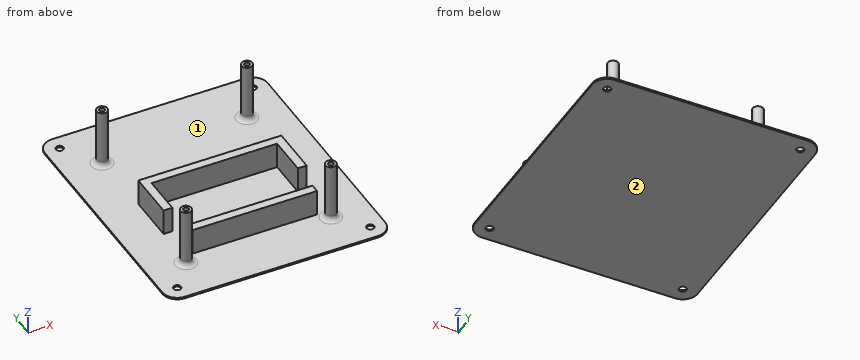
```python
from build123d import *

# Parameters (mm, degrees)
BASE_FLANGE1_DEPTH      = 1
SKETCH7_R               = 2.125
CUT_EXTRUDE1_DEPTH      = 10
SKETCH8_R               = 3
BOSS_EXTRUDE3_DEPTH     = 34
EXTRUDE_THIN1_OUTLINE_W = 71
EXTRUDE_THIN1_OUTLINE_H = 5
EXTRUDE_THIN1_DEPTH     = 15
SKETCH17_R              = 1.5
CUT_EXTRUDE3_DEPTH      = 13
SKETCH15_R              = 1.5
CUT_EXTRUDE4_DEPTH      = 13
SKETCH13_R              = 1.5
CUT_EXTRUDE5_DEPTH      = 13
SKETCH14_R              = 1.5
CUT_EXTRUDE6_DEPTH      = 13
FILLET1_R               = 3
FILLET2_R               = 3
FILLET3_R               = 3
FILLET4_R               = 3


# Read off the part's stored shape, not the designer's step: Extrude-Thin1
# Sheet-metal steps are written as plain solids
with BuildPart() as part:
    # Sketch1 → Base-Flange1 (new body)
    with BuildSketch(Plane.XY):
        with BuildLine():
            Line((-55.005, -73.465), (55.005, -73.465))
            ThreePointArc((55.005, -73.465), (60.987123369, -70.987123369), (63.465, -65.005))
            Line((63.465, -65.005), (63.465, 65.005))
            ThreePointArc((63.465, 65.005), (60.987123369, 70.987123369), (55.005, 73.465))
            Line((55.005, 73.465), (-55.005, 73.465))
            ThreePointArc((-55.005, 73.465), (-60.987123369, 70.987123369), (-63.465, 65.005))
            Line((-63.465, 65.005), (-63.465, -65.005))
            ThreePointArc((-63.465, -65.005), (-60.987123369, -70.987123369), (-55.005, -73.465))
        make_face()
    extrude(amount=-BASE_FLANGE1_DEPTH)

    # Sketch7 → Cut-Extrude1 (cut)
    with BuildSketch(Plane(origin=(0, 0, -1), x_dir=(-1, 0, 0), z_dir=(0, 0, -1))):
        with Locations((55.005, 65.005)):
            Circle(SKETCH7_R)
        with Locations((-55.005, 65.005)):
            Circle(SKETCH7_R)
        with Locations((55.005, -65.005)):
            Circle(SKETCH7_R)
        with Locations((-55.005, -65.005)):
            Circle(SKETCH7_R)
    extrude(amount=-CUT_EXTRUDE1_DEPTH, mode=Mode.SUBTRACT)

    # Sketch8 → Boss-Extrude3 (add)
    with BuildSketch(Plane.XY):
        with Locations((-41.5, -48.465)):
            Circle(SKETCH8_R)
        with Locations((-41.5, 44.372)):
            Circle(SKETCH8_R)
        with Locations((41.05, -48.465)):
            Circle(SKETCH8_R)
        with Locations((41.05, 44.372)):
            Circle(SKETCH8_R)
    extrude(amount=BOSS_EXTRUDE3_DEPTH)

    # Extrude-Thin1 outline → Extrude-Thin1 (add)
    with BuildSketch(Plane.XY):
        with Locations((0.25, -40.965)):
            Rectangle(EXTRUDE_THIN1_OUTLINE_W, EXTRUDE_THIN1_OUTLINE_H)
        Polygon((-40.75, 5.735), (-40.75, -22.265), (-35.75, -22.265), (-35.75, 0.735), (35.75, 0.735), (35.75, -22.265), (40.75, -22.265), (40.75, 5.735), align=None)
    extrude(amount=EXTRUDE_THIN1_DEPTH)

    # Sketch17 → Cut-Extrude3 (cut)
    with BuildSketch(Plane.XY.offset(34)):
        with Locations((41.05, -48.465)):
            Circle(SKETCH17_R)
    extrude(amount=-CUT_EXTRUDE3_DEPTH, mode=Mode.SUBTRACT)

    # Sketch15 → Cut-Extrude4 (cut)
    with BuildSketch(Plane.XY.offset(34)):
        with Locations((-41.5, -48.465)):
            Circle(SKETCH15_R)
    extrude(amount=-CUT_EXTRUDE4_DEPTH, mode=Mode.SUBTRACT)

    # Sketch13 → Cut-Extrude5 (cut)
    with BuildSketch(Plane.XY.offset(34)):
        with Locations((-41.5, 44.372)):
            Circle(SKETCH13_R)
    extrude(amount=-CUT_EXTRUDE5_DEPTH, mode=Mode.SUBTRACT)

    # Sketch14 → Cut-Extrude6 (cut)
    with BuildSketch(Plane.XY.offset(34)):
        with Locations((41.05, 44.372)):
            Circle(SKETCH14_R)
    extrude(amount=-CUT_EXTRUDE6_DEPTH, mode=Mode.SUBTRACT)

    # Fillet1
    fillet1_edges = [part.edges().sort_by_distance(p)[0] for p in [
        (-44.5, -48.465, 0),
    ]]
    fillet(fillet1_edges, radius=FILLET1_R)

    # Fillet2
    fillet2_edges = [part.edges().sort_by_distance(p)[0] for p in [
        (38.05, -48.465, 0),
    ]]
    fillet(fillet2_edges, radius=FILLET2_R)

    # Fillet3
    fillet3_edges = [part.edges().sort_by_distance(p)[0] for p in [
        (-44.5, 44.372, 0),
    ]]
    fillet(fillet3_edges, radius=FILLET3_R)

    # Fillet4
    fillet4_edges = [part.edges().sort_by_distance(p)[0] for p in [
        (38.05, 44.372, 0),
    ]]
    fillet(fillet4_edges, radius=FILLET4_R)


solid = part.part
```
Here's how the part is built. I have some questions about the finished solid (model axes, mm). Face numbers are marked on the shaded views. Give positions to 0.01 mm unless a question says otherwise; leave off trailing zeros. Order: outer loops, then holes, each group sorted by start corner. A loop starts at its lowest first (then second) coordinate and runs counter-clockwise, first axis right, second up. Notation, with made-up numbers: (12.5, 23.5) - (36.5, 23.5) arc R8 ccw to (36.5, 37.5) - close; hole circle Ø8 at (66.5, 7.25). An arc over 180 degrees is marked (long way). Answer as a JSON object with one key per item and string values. Group by question number.
Item 1: If we section it at B-B on y = -9: Please give me the cut outline in (x, z) (3 decimals).
Item 2: If we section it at A-A on z = 24.5: Please give me the cut outline in (x, y) (3 decimals).
Item 3: For P1, Ø0.9, axis at x = 41.5, y = 44, coming from the +Z side; P2, Ø7.5, axis at x = -14.5, z = 5, coming from the +Y side (3 decimals); P3, Ø12, axis at x = 19.5, y = 29.5, coming from the +Z side, each with a flat end and sliding along its axis, tell me the tip position at first contact or that it passes through.
Item 4: If we section it at D-D on y = -28.5: Please give me the cut outline in (x, z) (3 decimals).
Item 5: If we section it at C-C on z = 12.5: Please give me the cut outline in (x, y) (3 decimals).
Item 6: Please list where these lines run through material, in increasing order: probe 1 along Y at (x, z) = (41.05, 30) (3 decimals); probe 2 along Y at (x, z) = (-19.5, 14) (3 decimals); probe 3 along Z at (x, y) = (-14.5, 52.5).
Item 7: If we mould it in two halves opening along X, with no side actions, what happens to the marked faces 1 and 2? For each: pulls with the +X half, pulls with the -X half, needs draft (parallel to the pull), parting line crosses it, or undercut.
Result set:
{
 "1": {"outline": "(-63.465, -1) - (63.465, -1) - (63.465, 0) - (40.75, 0) - (40.75, 15) - (35.75, 15) - (35.75, 0) - (-35.75, 0) - (-35.75, 15) - (-40.75, 15) - (-40.75, 0) - (-63.465, 0) - close"},
 "2": {"outline": "circle Ø6 at (-41.5, -48.465); circle Ø6 at (-41.5, 44.372); circle Ø6 at (41.05, -48.465); circle Ø6 at (41.05, 44.372); hole circle Ø3 at (-41.5, -48.465); hole circle Ø3 at (-41.5, 44.372); hole circle Ø3 at (41.05, -48.465); hole circle Ø3 at (41.05, 44.372)"},
 "3": {"P1": "z = 21", "P2": "y = 5.735", "P3": "z = 0"},
 "4": {"outline": "(-63.465, -1) - (63.465, -1) - (63.465, 0) - (-63.465, 0) - close"},
 "5": {"outline": "circle Ø6 at (-41.5, -48.465); circle Ø6 at (-41.5, 44.372); (-40.75, -22.265) - (-35.75, -22.265) - (-35.75, 0.735) - (35.75, 0.735) - (35.75, -22.265) - (40.75, -22.265) - (40.75, 5.735) - (-40.75, 5.735) - close; (-35.25, -43.465) - (35.75, -43.465) - (35.75, -38.465) - (-35.25, -38.465) - close; circle Ø6 at (41.05, -48.465); circle Ø6 at (41.05, 44.372)"},
 "6": {"probe 1": "-51.465 to -49.965, -46.965 to -45.465, 41.372 to 42.872, 45.872 to 47.372", "probe 2": "-43.465 to -38.465, 0.735 to 5.735", "probe 3": "-1 to 0"},
 "7": {"face 1": "undercut", "face 2": "needs draft"}
}
